```python
from build123d import *

# Parameters (mm, degrees)
SKETCH1_R           = 5
BOSS_EXTRUDE1_DEPTH = 10
SKETCH2_R           = 3
BOSS_EXTRUDE2_DEPTH = 5
SKETCH3_R           = 3
CUT_EXTRUDE1_DEPTH  = 5
SKETCH4_W           = 4
SKETCH4_H           = 4
BOSS_EXTRUDE3_DEPTH = 8
CIRPATTERN1_COUNT   = 2
CIRPATTERN1_ANGLE   = 90


with BuildPart() as part:
    # Sketch1 → Boss-Extrude1 (new body)
    with BuildSketch(Plane(origin=(0, 0, 0), x_dir=(1, 0, 0), z_dir=(0, 1, 0))):
        with Locations(Location((0, 0, 0), (0, 0, 270))):
            Circle(SKETCH1_R)
    extrude(amount=BOSS_EXTRUDE1_DEPTH)

    # Sketch2 → Boss-Extrude2 (add)
    with BuildSketch(Plane(origin=(0, 10, 0), x_dir=(1, 0, 0), z_dir=(0, 1, 0))):
        with Locations(Location((0, 0, 0), (0, 0, 270))):
            Circle(SKETCH2_R)
    extrude(amount=BOSS_EXTRUDE2_DEPTH)

    # Sketch3 → Cut-Extrude1 (cut)
    with BuildSketch(Plane.XZ):
        with Locations(Location((0, 0, 0), (0, 0, 90))):
            Circle(SKETCH3_R)
    extrude(amount=-CUT_EXTRUDE1_DEPTH, mode=Mode.SUBTRACT)

    # Sketch4 → Boss-Extrude3 (add)
    with BuildSketch(Plane.XY):
        with Locations((0.169651393, 12.969101694)):
            Rectangle(SKETCH4_W, SKETCH4_H)
    boss_extrude3 = extrude(amount=BOSS_EXTRUDE3_DEPTH)

    # CirPattern1: Boss-Extrude3 ×2 about axis
    cirpattern1_axis = Axis((0, 0, 0), (0, 1, 0))
    for i in range(1, CIRPATTERN1_COUNT):
        add(boss_extrude3.rotate(cirpattern1_axis, i * CIRPATTERN1_ANGLE / (CIRPATTERN1_COUNT - 1)))


solid = part.part
```
Geometry check sheet. Reference: the model listing, model coordinates, mm. A direction names the side the tool comes from. Coordinates: 2 decimals unless noted, no trailing zeros. Write each loop counter-clockwise with the first axis right and the second up, starting at its lowest first coordinate (ties: lowest second). Pieces come first, ordered by that corner, then holes. Notation, with made-up numbers: (83, 70.25) -> (104, 70.25) arc R29 cw to (104, 98.25) -> close; hole circle Ø11 at (-4.75, -39). An arc over 180 degrees is marked (long way). Use CSV: the item, a comma, the result in double quotes. Start each with the question number.
Item 1: Mould release check, pull along Z, two halves, no side actions. Record for faces 1 (the flat face through (5, 13, 1.83)), 2 (the flat face through (0, 5, 0)), 3 (the cylindrical face through (-4.88, 4.93, -1.08)): released by +Z, released by -Z, zero draft, split by the parting line, or undercut.
Item 2: Set-up check for faces 4 (the flat face through (2.17, 13, 5)), 5 (the cylindrical face through (-1.8, 11.9, -2.4)), 6 (the cylindrical face through (-0.9, 2.46, 2.86)): record each of +Z, -Z, +X, -X, +Y, -Y from which the full face is reachable in a straight line by a thin tool's end or side.
Item 3: Thickness scan on line 1 (X direction, y = 2.95, z = 0); line 2 (Y direction, x = -1.5, z = -2); line 3 (Y direction, x = 1.25, z = 3.25). Record the ranges inside material, lowest first.
Item 4: Cross-section at C-C, the plane y = 13. Record the cut outline in (x, z), plus the area to 3 significant figures.
Item 5: Cross-section at D-D, the plane y = 4.5. Record the cut outline in (x, z).
Item 6: Depth check by flat-ended pin: pin 1 Ø2 at (x, y) = (4, 4) entering from -Z; pin 2 Ø3 at (x, y) = (4.5, 12.5) entering from +Z; pin 3 Ø3 at (x, z) = (-0.5, 6) entering from +Y. Enter the tip coordinate at first touch or a pass-through.
Answers:
1,face 1,"released by +Z"
1,face 2,"undercut"
1,face 3,"split by the parting line"
2,face 4,"+Z, +X, +Y"
2,face 5,"none"
2,face 6,"-Y"
3,line 1,"-5 to -3, 3 to 5"
3,line 2,"5 to 15"
3,line 3,"0 to 10, 10.97 to 14.97"
4,outline,"(-1.83, 2.38) arc R3 ccw (long way) to (2.07, -2.17) -> (8, -2.17) -> (8, 1.83) -> (2.38, 1.83) arc R3 ccw to (2.17, 2.07) -> (2.17, 8) -> (-1.83, 8) -> close"
4,area,"70.2 mm^2"
5,outline,"circle Ø10 at (0, 0); hole circle Ø6 at (0, 0)"
6,pin 1,"z = -4"
6,pin 2,"z = 1.83"
6,pin 3,"y = 14.97"
